Geometry check sheet. Reference: drawing and pictorial views, mm from the part's lowest x, y, z. A direction names the side the tool comes from. Coordinates: 2 decimals unless noted, no trailing zeros. Loops run counter-clockwise (first coordinate to the right, second up) from the corner with the lowest first, then second, coordinate; pieces in that order, holes last. Notation, with made-up numbers: (18, 26.25) -> (44, 26.25) arc R10 cw to (44, 37.25) -> close; hole circle Ø9 at (70, -21.5). An arc over 180 degrees is marked (long way). Answer as a JSON object with one key per item and string values.
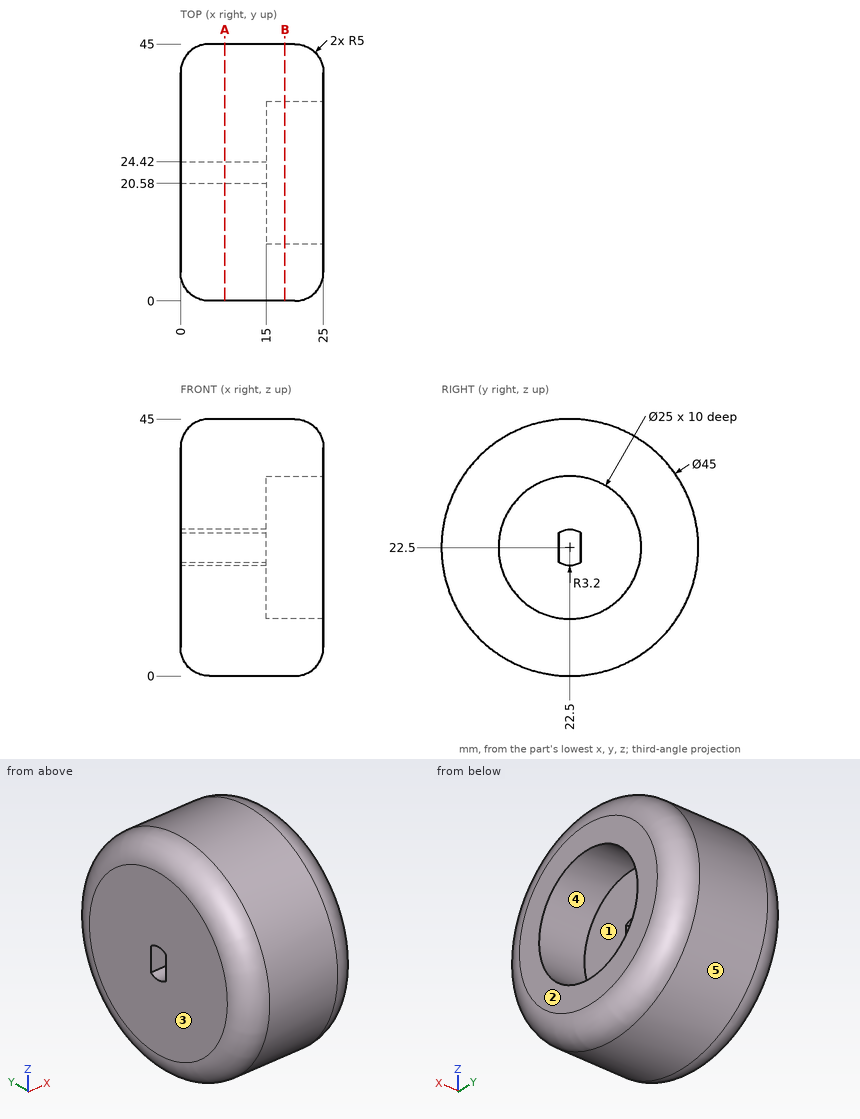
1. Tool access check on the marked faces 1 and 2. Record the directions out of +Z, -Z, +X, -X, +Y, -Y that give a thin tool (end or side, any length) a straight path to the whole face; none if there is none.
Evaluation:
{"face 1": "+X", "face 2": "+Z, -Z, +X, +Y, -Y"}
2. Thickness scan on probe 1 along Y at (x, z) = (12.75, 23); probe 2 along Y at (x, z) = (18, 22.5); probe 3 along X at (y, z) = (26, 18.5). Record the ranges inside material, lowest first. Write a range as from..to.
Evaluation:
{"probe 1": "y = 0.01..20.58, 24.42..44.99", "probe 2": "y = 0..10, 35..45", "probe 3": "x = 0..15"}
3. Mould release check, pull along Y, two halves, no side actions. Record for the marked faces 3, 4 and 5: released by +Y, released by -Y, zero draft, split by the parting line, or undercut.
Evaluation:
{"face 3": "zero draft", "face 4": "undercut", "face 5": "split by the parting line"}
4. Section check A-A, the plane x = 7.75. Record the boundary of the cut face in (y, z).
Evaluation:
{"outline": "circle Ø45 at (22.5, 22.5); hole (20.58, 19.94) arc R3.2 ccw to (24.42, 19.94) -> (24.42, 25.06) arc R3.2 ccw to (20.58, 25.06) -> close"}
5. Section check B-B, the plane x = 18.25. Record the boundary of the cut face in (y, z).
Evaluation:
{"outline": "circle Ø45 at (22.5, 22.5); hole circle Ø25 at (22.5, 22.5)"}
6. Depth check by flat-ended pin: P1, Ø1.5, axis at x = 18, y = 37.5, coming from the -Z side; P2, Ø1, axis at x = 10, z = 24.5, coming from the -Y side; P3, Ø2, axis at x = 11, z = 37, coming from the -Y side; P4, Ø6, axis at y = 17, z = 40, coming from the +X side. Enter the tip coordinate at first touch or a pass-through.
Evaluation:
{"P1": "stops at z = 5.09", "P2": "stops at y = 0.05", "P3": "stops at y = 4.5", "P4": "stops at x = 25"}
